from build123d import *

# Parameters (mm, degrees)
F0_R      = 12.7
F1_DEPTH  = 76.2
F2_R      = 38.09999
F3_R      = 19.05
F4_DEPTH  = 50.801
F6_DEPTH  = 76.201
F8_DEPTH  = 50.801
F11_DEPTH = 50.801


# Not quite as in the source:
# - a fillet or chamfer is up to 0.001 mm smaller than in the source, because OpenCascade refuses the exact size


with BuildPart() as f1:
    # F0 (on Top) → F1 (new body)
    with BuildSketch(Plane.XY):
        with BuildLine():
            Line((25.4, -152.4), (25.4, 0))
            ThreePointArc((25.4, 0), (0, 25.4), (-25.4, 0))
            Line((-25.4, 0), (-25.4, -152.4))
            Line((-25.4, -152.4), (25.4, -152.4))
        make_face()
        Circle(F0_R, mode=Mode.SUBTRACT)
    extrude(amount=F1_DEPTH)

    # F2 (radius 38.1 in the source; OpenCascade refuses exactly that, so slightly less here)
    f2_edges = [f1.edges().sort_by_distance(p)[0] for p in [
        (0, -152.4, 76.2),
        (0, -152.4, 0),
    ]]
    fillet(f2_edges, radius=F2_R)

    # F3 (on face) → F4 (cut, through all)
    with BuildSketch(Plane.YZ.offset(25.4)):
        with Locations((-121.2292984128, 38.5233350098)):
            Circle(F3_R)
    extrude(amount=-F4_DEPTH, mode=Mode.SUBTRACT)

    # F5 (on face) → F6 (cut, through all)
    with BuildSketch(Plane.XY.offset(76.2)):
        with BuildLine():
            Line((-5.7387360482, -29.3549266663), (-5.6882195357, -68.4034783226))
            ThreePointArc((-5.6882195357, -68.4034783226), (0.0700403354, -77.5756190124), (5.6245744634, -68.2786909069))
            Line((5.6245744634, -68.2786909069), (5.5746364254, -29.6772918832))
            ThreePointArc((5.5746364254, -29.6772918832), (0.1808646036, -20.2891562763), (-5.7387360482, -29.3549266663))
        make_face()
    extrude(amount=-F6_DEPTH, mode=Mode.SUBTRACT)

    # F7 (on face) → F8 (cut, through all)
    with BuildSketch(Plane(origin=(-25.4, 0, 0), x_dir=(0, -1, 0), z_dir=(-1, 0, 0))):
        Polygon((0, 63.5), (0, 12.7), (12.9918251187, 12.7), (46.0542105138, 12.633157894), (46.0542105138, 63.5), (12.9918251187, 63.5), align=None)
    extrude(amount=-F8_DEPTH, mode=Mode.SUBTRACT)

    # F10 (on offset) → F11 (cut, through all)
    with BuildSketch(Plane.YZ.offset(25.4)):
        Polygon((25.4299268126, 63.3701309562), (0, 63.3701309562), (0, 12.7395335585), (25.4423227161, 12.7395335585), align=None)
    extrude(amount=-F11_DEPTH, mode=Mode.SUBTRACT)


solid = f1.part
Geometry check sheet. Reference: the model listing, model coordinates, mm. A direction names the side the tool comes from. Round coordinates to 2 decimals unless told otherwise and drop trailing zeros. Loops run counter-clockwise (first coordinate to the right, second up) from the corner with the lowest first, then second, coordinate; pieces in that order, holes last. Notation, with made-up numbers: (50, -12.5) -> (89, -12.5) arc R30 cw to (89, 19.5) -> close; hole circle Ø3 at (86, 57). An arc over 180 degrees is marked (long way). Answer as a JSON object with one key per item and string values. Group by question number.
Item 1: Thickness scan on line 1 along Z through (x, y) = (-9, -17); line 2 along Z through (x, y) = (14.5, 9.5); line 3 along X through (y, z) = (-57, 56.5). Record the ranges inside material, lowest first.
Item 2: Set-up check for faces 4 (the face through (0.36, -141.54, 11.46)), 5 (the face through (0, 13, 63.37)), 6 (the face through (-6, -23, 63.5)): record each of +Z, -Z, +X, -X, +Y, -Y from which the full face is reachable in a straight line by a thin tool's end or side.
Item 3: Cross-section at B-B, the plane z = 55. Record the cut outline in (x, y), plus the area to 3 significant figures.
Item 4: Cross-section at C-C, the plane y = -25.5. Record the cut outline in (x, z), plus the area to 3 significant figures.
Item 5: Release check for a two-part mould opening along Z. For faces 1 (the face through (-25.4, -75, 38)), 2 (the face through (-6, -12, 12.7)), 3 (the face through (-6, -43, 0)) record: pulls with the +Z half, pulls with the -Z half, needs draft (parallel to the pull), parting line crosses it, or undercut.
Item 6: Depth check by flat-ended pin: pin 1 Ø2 at (x, z) = (0, 60) entering from -Y; pin 2 Ø3 at (x, z) = (-17.5, 66) entering from +Y; pin 3 Ø21.5 at (x, z) = (-14, 38.5) entering from +Y. Enter the tip coordinate at first touch or a pass-through.
Item 7: Cross-section at A-A, the plane x = 0. Count the separate pieces of the cut face and the enclosed holes in it, plus the area to 3 significant figures.
Determined:
{
 "1": {"line 1": "z = 0 to 12.69, 63.5 to 76.2", "line 2": "z = 0 to 12.74, 63.37 to 76.2", "line 3": "x = -25.4 to -5.7, 5.61 to 25.4"},
 "2": {"face 4": "-Z, +X, -X, -Y", "face 5": "+X, -X, +Y", "face 6": "+X, -X"},
 "3": {"outline": "(-25.4, -148.45) -> (25.4, -148.45) -> (25.4, -130.79) -> (-25.4, -130.79) -> close; (-25.4, -111.67) -> (25.4, -111.67) -> (25.4, -46.05) -> (5.6, -46.05) -> (5.62, -68.28) arc R6.35 cw (long way) to (-5.69, -68.4) -> (-5.72, -46.05) -> (-25.4, -46.05) -> close", "area": "3,880 mm²"},
 "4": {"outline": "(-25.4, 0) -> (-6.25, 0) -> (-6.25, 12.67) -> (-25.4, 12.67) -> close; (-25.4, 63.5) -> (-6.25, 63.5) -> (-6.25, 76.2) -> (-25.4, 76.2) -> close; (6.25, 0) -> (25.4, 0) -> (25.4, 12.67) -> (6.25, 12.67) -> close; (6.25, 63.5) -> (25.4, 63.5) -> (25.4, 76.2) -> (6.25, 76.2) -> close", "area": "972 mm²"},
 "5": {"face 1": "needs draft", "face 2": "undercut", "face 3": "pulls with the -Z half"},
 "6": {"pin 1": "stops at y = -146.16", "pin 2": "stops at y = 19.73", "pin 3": "stops at y = -46.05"},
 "7": {"separate pieces": "5", "enclosed holes": "1", "area": "4,460 mm²"}
}
